The listing builds one solid part. Answer for the finished solid, in the listing's coordinates (mm). A direction names the side the tool comes from. Give positions to 0.01 mm unless a question says otherwise; leave off trailing zeros. Write each loop counter-clockwise with the first axis right and the second up, starting at its lowest first coordinate (ties: lowest second). Pieces come first, ordered by that corner, then holes. Notation, with made-up numbers: (64.25, 0) - (86.25, 0) arc R19 ccw to (86.25, 4) - close; hole circle Ø7 at (-14, -14.75). An arc over 180 degrees is marked (long way). One line per question, with ' | ' between items. Start each with the question number.
1. The mould has two halves that part along X. Classify faces 5 (the face through (7.52, 34.02, -7.55)), 6 (the face through (3.53, 35.94, -9.48)), 7 (the face through (13.163, 19.505, -9.481)): +X half, -X half, draft (parallel to the pull), parting line (faces both ways), or undercut.
2. A cutting plane is placed at A-A (z = -11.25). Determine the outline of the cut face in (x, y).
3. For faces 1 (the face through (6.53, 19.54, -1.25)), 2 (the face through (-1.4, 27.7, -6.35)), 3 (the face through (13.06, 36, -9.48)), 4 (the face through (3.638, 19.444, -9.481)), determine the directions among +Z, -Z, +X, -X, +Y, -Y from which every point of the face is accessible in a straight line to the end or side of a thin tool.
4. Find the intervals of material crossed by L1, parallel to X at y = 27.75, z = -3.5; L2, parallel to Z at x = 18.25, y = 27, in increasing order. Write a range as from..to.
5. Given P1, Ø2, axis at y = 23, z = -11, coming from the +X side; P2, Ø1, axis at y = 37, z = -4.5, coming from the +X side; P3, Ø1.5, axis at x = 11, y = 38, coming from the +Z side; P4, Ø1.5, axis at x = 4, y = 32.5, coming from the +Z side, each flat-ended and moving along its own axis, determine where each tip first touches the part or whether it passes through.
```python
from build123d import *
from build123d.topology import SkipClean

# Parameters (mm, degrees)
SKETCH3_R           = 14.9225
BOSS_EXTRUDE1_DEPTH = 12.7
SKETCH11_R          = 6.35
CUT_EXTRUDE3_DEPTH  = 12.7
SKETCH12_R          = 8.382
CUT_EXTRUDE4_DEPTH  = 2.54
THREAD1_PITCH       = 1.5875
CUT_EXTRUDE6_START  = -6.35
SKETCH14_R          = 14.9225
CUT_EXTRUDE6_DEPTH  = 6.35


with BuildPart() as part:
    # Sketch3 → Boss-Extrude1 (new body)
    with BuildSketch(Plane.XY):
        with Locations((8.347593151, 27.723781851)):
            Circle(SKETCH3_R)
    extrude(amount=-BOSS_EXTRUDE1_DEPTH)

    # Sketch11 → Cut-Extrude3 (cut)
    with BuildSketch(Plane.XY):
        with Locations((8.347593151, 27.723781851)):
            Circle(SKETCH11_R)
    extrude(amount=-CUT_EXTRUDE3_DEPTH, mode=Mode.SUBTRACT)

    # Sketch12 → Cut-Extrude4 (cut)
    with BuildSketch(Plane.XY):
        with Locations((8.347593151, 27.723781851)):
            Circle(SKETCH12_R)
    extrude(amount=-CUT_EXTRUDE4_DEPTH, mode=Mode.SUBTRACT)

    # Thread1: the profile of Thread Profile1 profile screwed along a right-hand helix of 4.8 turns, 8 arcs to a turn; built about Z, then put on its axis
    thread1_z = Axis((0, 0, 0), (0, 0, 1))
    thread1_corners = [(14.9228, 0, -0.000173205), (14.9228, 0, 0.694704453), (14.492870212, 0, 0.446484374), (14.492870212, 0, 0.248046874)]
    with BuildLine(mode=Mode.PRIVATE) as thread1_profile:
        Line(thread1_corners[0], thread1_corners[1])
        Line(thread1_corners[1], thread1_corners[2])
        Line(thread1_corners[2], thread1_corners[3])
        Line(thread1_corners[3], thread1_corners[0])
    thread1_cap = Face(thread1_profile.wire())
    thread1_turn_angles = [0, 22.5, 45, 67.5, 90, 112.5, 135, 157.5, 180, 202.5, 225, 247.5, 270, 292.5, 315, 337.5, 360]
    thread1_turn_weights = [1, 0.9238795325112867, 1, 0.9238795325112867, 1, 0.9238795325112867, 1, 0.9238795325112867, 1, 0.9238795325112867, 1, 0.9238795325112867, 1, 0.9238795325112867, 1, 0.9238795325112867, 1]
    thread1_turn_rails = [Edge.make_bspline([Vector(p[0], p[1], 0).rotate(thread1_z, thread1_turn_angles[k]) / thread1_turn_weights[k] + Vector(0, 0, p[2] + THREAD1_PITCH * thread1_turn_angles[k] / 360) for k in range(17)], [0, 0, 0, 1, 1, 2, 2, 3, 3, 4, 4, 5, 5, 6, 6, 7, 7, 8, 8, 8], 2, thread1_turn_weights) for p in thread1_corners]
    thread1_turn_sides = [Face.make_surface_from_curves(thread1_turn_rails[p[0]], thread1_turn_rails[p[1]]) for p in [(0, 1), (1, 2), (2, 3), (3, 0)]]
    thread1_last_angles = [1440, 1462.5, 1485, 1507.5, 1530, 1552.5, 1575, 1597.5, 1620, 1642.5, 1665, 1687.5, 1710, 1719, 1728]
    thread1_last_weights = [1, 0.9238795325112867, 1, 0.9238795325112867, 1, 0.9238795325112867, 1, 0.9238795325112867, 1, 0.9238795325112867, 1, 0.9238795325112867, 1, 0.9876883405951378, 1]
    thread1_last_rails = [Edge.make_bspline([Vector(p[0], p[1], 0).rotate(thread1_z, thread1_last_angles[k]) / thread1_last_weights[k] + Vector(0, 0, p[2] + THREAD1_PITCH * thread1_last_angles[k] / 360) for k in range(15)], [0, 0, 0, 1, 1, 2, 2, 3, 3, 4, 4, 5, 5, 6, 6, 7, 7, 7], 2, thread1_last_weights) for p in thread1_corners]
    thread1_last_sides = [Face.make_surface_from_curves(thread1_last_rails[p[0]], thread1_last_rails[p[1]]) for p in [(0, 1), (1, 2), (2, 3), (3, 0)]]
    thread1 = Plane(origin=(8.347593151, 27.723781851, 0.79375), x_dir=(-1, 0, 0), z_dir=(0, 0, -1)) * Solid(Shell([*[p.moved(Location((0, 0, THREAD1_PITCH * i))) for i in range(4) for p in thread1_turn_sides], *thread1_last_sides, thread1_cap, thread1_cap.rotate(thread1_z, 1728).moved(Location((0, 0, THREAD1_PITCH * 1728 / 360)))]))
    add(thread1, mode=Mode.SUBTRACT)

    # Sketch14 → Cut-Extrude6 (cut)
    with SkipClean():  # the faces are left unmerged after this step: merging them gives an invalid solid
        with BuildSketch(Plane(origin=(0, 0, -12.7), x_dir=(-1, 0, 0), z_dir=(0, 0, -1)).offset(CUT_EXTRUDE6_START)):
            with Locations((-8.347593151, 27.723781851)):
                Circle(SKETCH14_R)
            Polygon((1.186658464, 22.240576024), (1.168128197, 33.239083042), (-8.366123418, 38.722288869), (-17.881844766, 33.206987678), (-17.863314499, 22.20848066), (-8.329062884, 16.725274833), align=None, mode=Mode.SUBTRACT)
        extrude(amount=CUT_EXTRUDE6_DEPTH, mode=Mode.SUBTRACT)
    add(part.part.scale(1), mode=Mode.REPLACE)  # the faces are merged on a copy


solid = part.part
```
Determined:
1) face 5: undercut | face 6: -X half | face 7: +X half
2) outline: (-1.19, 22.24) - (8.33, 16.73) - (17.86, 22.21) - (17.88, 33.21) - (8.37, 38.72) - (-1.17, 33.24) - close; hole circle Ø12.7 at (8.35, 27.72)
3) face 1: +Z | face 2: -Z | face 3: -Z, +X, +Y | face 4: -Z, -X, -Y
4) L1: -6.57..2, 14.7..22.84 | L2: -6.35..0
5) P1: x = 17.87 | P2: x = 20.42 | P3: z = 0 | P4: z = -2.54
